from build123d import *

# Parameters (mm, degrees)
F1_DEPTH = 6.35


with BuildPart() as f1:
    # F0 (on Front) → F1 (new body)
    with BuildSketch(Plane.XZ):
        with BuildLine():
            add(Edge.make_bspline(
                [(-69.2670494318, 19.05), (-67.3128640728, 16.2248080447), (-60.969426566, 13.3476320625), (-22.1680297811, 9.7510011569), (12.7, 12.1750152693)],
                knots=[0, 0, 0, 0, 0.2505960164, 1, 1, 1, 1], degree=3))
            ThreePointArc((-69.2670494318, 19.05), (-97.6377356755, 11.397017146), (-127, 10.2474875748))
            ThreePointArc((-127, 10.2474875748), (-100.6736295618, -10.1512932616), (-68.58, -19.05))
            ThreePointArc((-68.58, -19.05), (-30.48, -11.7126104241), (7.62, -19.05))
            Line((7.62, -19.05), (12.7, -19.05))
            ThreePointArc((12.7, -19.05), (27.4012824935, -6.4499702137), (46.4045489641, -10.16))
            ThreePointArc((46.4045489641, -10.16), (76.642998398, -12.2201918698), (106.172, -19.05))
            ThreePointArc((106.172, -19.05), (118.4151863409, -11.5249103993), (127, 0))
            ThreePointArc((127, 0), (70.6277336889, 13.3889326164), (12.7, 12.1750152693))
        make_face()
    extrude(amount=F1_DEPTH)


solid = f1.part
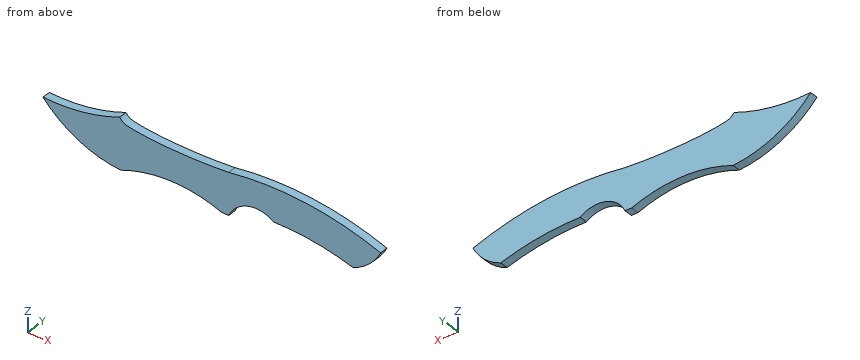
Part model, mm, in its own coordinate system. Give positions to 0.01 mm unless a question says otherwise; leave off trailing zeros. Loops run counter-clockwise (first coordinate to the right, second up) from the corner with the lowest first, then second, coordinate; pieces in that order, holes last. Notation, with made-up numbers: (18.5, 13) -> (52.5, 13) arc R34 cw to (52.5, 48) -> close; hole circle Ø2 at (-23.5, 11.25). An arc over 180 degrees is marked (long way). Write each question's results on one line, items separated by ' | '. Start each with the question number.
Q1. Band-saw the part on C-C on x = 22.5. List the corners of the cut face in (y, z), plus the area to 3 significant figures.
Q2. Pin check, flat tips, straight feed: P1, Ø1, axis at x = 83.5, y = -3, coming from the -Z side; P2, Ø1, axis at x = 28.5, y = -4, coming from the -Z side. Stop position of each tip, or through.
Q3. Band-saw the part on B-B on x = -85.5. List the corners of the cut face in (y, z), plus the area to 3 significant figures.
Q4. Wall check: L1, parallel to X at y = -2.75, z = -9.5; L2, parallel to X at y = -3, z = -3; L3, parallel to Z at x = 56, y = -3. Give the ranges that are in metal, low to high.
Q5. Band-saw the part on A-A on z = -15.5. List the corners of the cut face in (x, y), plus the area to 3 significant figures.
Results are:
1) outline: (-6.35, -8.39) -> (0, -8.39) -> (0, 13.42) -> (-6.35, 13.42) -> close | area: 138 mm²
2) P1: stops at z = -13.46 | P2: stops at z = -6.3
3) outline: (-6.35, -16.04) -> (0, -16.04) -> (0, 13.84) -> (-6.35, 13.84) -> close | area: 190 mm²
4) L1: x = -101.95 to 20.66, 45.48 to 120.47 | L2: x = -112.47 to 125.38 | L3: z = -10.29 to 14.47
5) outline: (-87.34, -6.35) -> (-58.1, -6.35) -> (-58.1, 0) -> (-87.34, 0) -> close; (-2.86, -6.35) -> (14.65, -6.35) -> (14.65, 0) -> (-2.86, 0) -> close; (93.46, -6.35) -> (113.24, -6.35) -> (113.24, 0) -> (93.46, 0) -> close | area: 423 mm²
